The model under review builds one solid part; all positions refer to its coordinate system, in mm. A direction names the side the tool comes from. Coordinates: 2 decimals unless noted, no trailing zeros. Order: outer loops, then holes, each group sorted by start corner. A loop starts at its lowest first (then second) coordinate and runs counter-clockwise, first axis right, second up. Notation, with made-up numbers: (-2, -5) -> (12, -5) arc R21 cw to (12, 16) -> close; hole circle Ø10 at (29, 68). An arc over 180 degrees is marked (long way). Put each result on its own line as item: value.
from build123d import *

# Parameters (mm, degrees)
ESBO_O1_R                = 11
RESSALTO_EXTRUS_O1_DEPTH = 5
ESBO_O3_R                = 1.25
CORTE_EXTRUS_O1_DEPTH    = 10.095971114
ESBO_O22_R               = 3
CORTE_EXTRUS_O6_DEPTH    = 5.5
ESBO_O23_R               = 3
CORTE_EXTRUS_O7_DEPTH    = 1.5
ESBO_O27_R               = 2
CORTE_EXTRUS_O8_DEPTH    = 10


# Read off the part's stored shape, not the designer's step: Broca de rosquear para tarraxa de M3x0.52
with BuildPart() as part:
    # Esboço1 → Ressalto-extrusão1 (new body)
    with BuildSketch(Plane(origin=(0, 0, 0), x_dir=(1, 0, 0), z_dir=(0, 1, 0))):
        with Locations(Location((0, 0, 0), (0, 0, 270))):
            Circle(ESBO_O1_R)
    extrude(amount=RESSALTO_EXTRUS_O1_DEPTH)

    # Esboço3 → Corte-extrusão1 (cut)
    with BuildSketch(Plane(origin=(0, 5, 0), x_dir=(1, 0, 0), z_dir=(0, 1, 0))):
        with Locations(Location((0, 7.7, 0), (0, 0, 270))):
            Circle(ESBO_O3_R)
        with Locations(Location((6.668395609, -3.85, 0), (0, 0, 270))):
            Circle(ESBO_O3_R)
        with Locations(Location((-6.668395609, -3.85, 0), (0, 0, 270))):
            Circle(ESBO_O3_R)
    extrude(amount=-CORTE_EXTRUS_O1_DEPTH, mode=Mode.SUBTRACT)

    # Esboço22 → Corte-extrusão6 (cut)
    with BuildSketch(Plane(origin=(0, 5, 0), x_dir=(1, 0, 0), z_dir=(0, 1, 0))):
        with Locations((-11.258330249, 6.5)):
            Circle(ESBO_O22_R)
        with Locations((0, -13)):
            Circle(ESBO_O22_R)
        with Locations((11.258330249, 6.5)):
            Circle(ESBO_O22_R)
    extrude(amount=-CORTE_EXTRUS_O6_DEPTH, mode=Mode.SUBTRACT)

    # Esboço23 → Corte-extrusão7 (cut)
    with BuildSketch(Plane(origin=(0, 0, 0), x_dir=(-1, 0, 0), z_dir=(0, -1, 0))):
        with Locations(Location((-6.668395609, -3.85, 0), (0, 0, 90))):
            Circle(ESBO_O23_R)
        with Locations(Location((6.668395609, -3.85, 0), (0, 0, 90))):
            Circle(ESBO_O23_R)
        with Locations(Location((0, 7.7, 0), (0, 0, 90))):
            Circle(ESBO_O23_R)
    extrude(amount=-CORTE_EXTRUS_O7_DEPTH, mode=Mode.SUBTRACT)

    # Esboço27 → Corte-extrusão8 (cut)
    with BuildSketch(Plane.XZ):
        with Locations(Location((0, 0, 0), (0, 0, 270))):
            Circle(ESBO_O27_R)
    extrude(amount=-CORTE_EXTRUS_O8_DEPTH, mode=Mode.SUBTRACT)

    # Broca de rosquear para tarraxa de M3 2 → Broca de rosquear para tarraxa de M3x0.52 (revolve, cut)
    with BuildSketch(Plane(origin=(0, 2.382860609, 0), x_dir=(0, 1, 0), z_dir=(0.11587924714300103, 0, -0.9932633085348372))):
        Polygon((0, -11.00002072), (1.275019909, -11.000019909), (1.249997575, -10.974997575), (1.25, -1.561025492), (0, -1.561025492), align=None)
    revolve(axis=Axis((0, 2.382860609, 0), (0.9932633085348372, 0, 0.11587924714300103)), mode=Mode.SUBTRACT)


solid = part.part
Item 1: For line 1 (X direction, y = 1.3, z = 2.25); line 2 (X direction, y = 3.5, z = 3.85); line 3 (Z direction, x = -0.5, y = 4.25), list the stretches that pass through material, from the lowest coordinate up. Write a range as from..to.
Answers below:
line 1: -10.77..-9.21, -4.13..4.13, 9.21..10.77
line 2: -10.3..-7.92, -5.42..5.42, 7.92..10.3
line 3: -10.99..-8.85, -6.55..-1.94, 1.94..10.04
Item 2: For faces 4 (the cylindrical face through (0.05, 3.27, -8.95)), 5 (the cylindrical face through (-4.139, 0.74, 2.237)), list the 3-axis set-ups (+Z, -Z, +X, -X, +Y, -Y) from which the entire face can be reached by the end or side of a thin tool; tool diameter is ignored.
Answers below:
face 4: +Y, -Y
face 5: -Y
Item 3: For pin 1 Ø3 at (x, z) = (0, -7.7) entering from -Y; pin 2 Ø1.5 at (x, y) = (8.5, 3) entering from +Z; pin 3 Ø3 at (y, z) = (3.5, 7) entering from -X; pin 4 Ø1.5 at (x, z) = (-6.67, 3.85) entering from +Y, all flat-tipped, find the tip position at first contact; note any pin that passes through.
Answers below:
pin 1: y = 1.5
pin 2: z = 7.81
pin 3: x = -9.53
pin 4: through
Item 4: Consider section C-C on x = 7.5. Write out the cut boundary in (y, z), and give its area (3 significant figures).
Answers below:
outline: (0, -8.05) -> (5, -8.05) -> (5, 2.92) -> (1.5, 2.92) -> (1.5, 0.97) -> (0, 0.97) -> close; (0, 6.73) -> (1.5, 6.73) -> (1.5, 4.78) -> (5, 4.78) -> (5, 8.05) -> (0, 8.05) -> close
area: 65.3 mm^2
Item 5: Consider section B-B on z = -8.5. Write out the cut boundary in (x, y).
Answers below:
outline: (-6.98, 0) -> (-2.89, 0) -> (-2.89, 1.5) -> (-0.96, 1.5) -> (-0.96, 5) -> (-6.98, 5) -> close; (0.96, 1.5) -> (2.89, 1.5) -> (2.89, 0) -> (6.98, 0) -> (6.98, 5) -> (0.96, 5) -> close
Item 6: Consider section D-D on z = 3.85. Write out the cut boundary in (x, y).
Answers below:
outline: (-10.3, 0) -> (-9.67, 0) -> (-9.67, 1.5) -> (-7.92, 1.5) -> (-7.92, 5) -> (-10.3, 5) -> close; (-5.42, 1.5) -> (-3.67, 1.5) -> (-3.67, 0) -> (3.67, 0) -> (3.67, 1.5) -> (5.42, 1.5) -> (5.42, 5) -> (-5.42, 5) -> close; (7.92, 1.5) -> (9.67, 1.5) -> (9.67, 0) -> (10.3, 0) -> (10.3, 5) -> (7.92, 5) -> close
Item 7: Consider section A-A on x = 0. Write out the cut boundary in (y, z), and give its area (4 significant figures).
Answers below:
outline: (0, -11) -> (5, -11) -> (5, -8.95) -> (1.5, -8.95) -> (1.5, -10.7) -> (0, -10.7) -> close; (0, -4.7) -> (1.5, -4.7) -> (1.5, -6.45) -> (5, -6.45) -> (5, -2) -> (0, -2) -> close; (0, 2) -> (5, 2) -> (5, 10) -> (0, 10) -> close
area: 67.25 mm^2
Item 8: Mouldability with a two-part tool opening along Z and no side actions: class faces 1 (the flat face through (5, 1.5, 4)), 2 (the cylindrical face through (0, 3, 10)), 3 (the cylindrical face through (9.46, 2.46, 5.61)) as +Z half, -Z half, draft (parallel to the pull), parting line (faces both ways), or undercut.
Answers below:
face 1: undercut
face 2: +Z half
face 3: parting line
